from build123d import *


with BuildPart() as part:
    # Sketch1 → Revolve1 (revolve)
    with BuildSketch(Plane.XY, mode=Mode.PRIVATE) as revolve1_sk:
        with BuildLine():
            Line((2.711324865, 30), (2.2, 30))
            Line((2.2, 30), (2.2, 28.9))
            Line((2.2, 28.9), (1.65, 28.582457352))
            Line((1.65, 28.582457352), (1.65, 20))
            Line((1.65, 20), (0, 19.008579979))
            Line((0, 19.008579979), (0, 0))
            ThreePointArc((0, 0), (1.347576341, 0.153288274), (2.626296799, 0.605320665))
            Line((2.626296799, 0.605320665), (3, 2))
            Line((3, 2), (3, 29.5))
            Line((3, 29.5), (2.711324865, 30))
        make_face()
    revolve(revolve1_sk.sketch.rotate(Axis((0, 30, 0), (0, -1, 0)), 90), axis=Axis((0, 30, 0), (0, -1, 0)))


solid = part.part
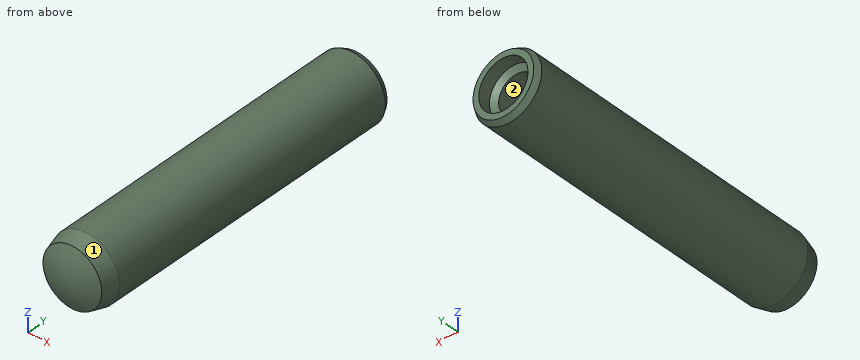
The listing builds one solid part. Answer for the finished solid, in the listing's coordinates (mm). Face numbers are marked on the shaded views. Coordinates: 2 decimals unless noted, no trailing zeros. Write each loop counter-clockwise with the first axis right and the second up, starting at its lowest first coordinate (ties: lowest second). Pieces come first, ordered by that corner, then holes. Notation, with made-up numbers: (-34, 20.5) -> (-11, 20.5) arc R15 ccw to (-11, 47.5) -> close; hole circle Ø6 at (14, -26). An arc over 180 degrees is marked (long way). One line per question, with ' | ' between items.
1. Section A-A (y = 13.25) is taken. Determine the outline of the cut face in (x, z).
Verdict:
outline: circle Ø6 at (0, 0)
2. For a pull along Z with two mould halves and no side action, classify the marked faces 1 and 2 as released by +Z, released by -Z, zero draft, split by the parting line, or undercut.
Verdict:
face 1: split by the parting line | face 2: undercut
3. Given pin 1 Ø1.5 at (x, y) = (0.5, 25.5) entering from -Z; pin 2 Ø1.5 at (x, z) = (-0.5, -1) entering from -Y; pin 3 Ø3 at (x, z) = (2, -2) entering from -Y, each flat-ended and moving along its own axis, determine where each tip first touches the part or whether it passes through.
Verdict:
pin 1: stops at z = -3 | pin 2: stops at y = 0.01 | pin 3: stops at y = 0.15
4. Section B-B (y = 21.75) is taken. Determine the outline of the cut face in (x, z).
Verdict:
outline: circle Ø6 at (0, 0); hole circle Ø3.3 at (0, 0)
5. Straight lines are drawn through the part: line 1 (X direction, y = 25.5, z = 0); line 2 (Z direction, x = -0.2, y = 16.5); line 3 (Z direction, x = 1.4, y = 20.5). For each, find the intervals that lie inside material, in ascending order.
Verdict:
line 1: x = -3 to -1.65, 1.65 to 3 | line 2: z = -2.99 to 2.99 | line 3: z = -2.65 to -0.87, 0.87 to 2.65
